Geometry: final body of the model. Coordinates: model frame, mm. A direction names the side the tool comes from. Give positions to 0.01 mm unless a question says otherwise; leave off trailing zeros. Order: outer loops, then holes, each group sorted by start corner. A loop starts at its lowest first (then second) coordinate and runs counter-clockwise, first axis right, second up. Notation, with made-up numbers: (42, -27.5) -> (66, -27.5) arc R35 ccw to (66, 10.5) -> close; hole circle Ø11 at (-1, 56.25). An arc over 180 degrees is marked (long way). One line per question, with ' | ' between items.
from build123d import *

# Parameters (mm, degrees)
BOSS_EXTRUDE1_DEPTH = 6.5
SKETCH2_R           = 12.5
BOSS_EXTRUDE2_DEPTH = 10.668
SKETCH3_R           = 10.5
BOSS_EXTRUDE3_DEPTH = 7
SKETCH4_R           = 7
BOSS_EXTRUDE4_DEPTH = 3


with BuildPart() as part:
    # Sketch1 → Boss-Extrude1 (new body)
    with BuildSketch(Plane.XY):
        with BuildLine():
            Line((-20.845394737, 3.828448545), (-5.427631579, 11.260142781))
            ThreePointArc((-5.427631579, 11.260142781), (0, 12.5), (5.427631579, 11.260142781))
            Line((5.427631579, 11.260142781), (20.845394737, 3.828448545))
            ThreePointArc((20.845394737, 3.828448545), (23.25, 0), (20.845394737, -3.828448545))
            Line((20.845394737, -3.828448545), (5.427631579, -11.260142781))
            ThreePointArc((5.427631579, -11.260142781), (0, -12.5), (-5.427631579, -11.260142781))
            Line((-5.427631579, -11.260142781), (-20.845394737, -3.828448545))
            ThreePointArc((-20.845394737, -3.828448545), (-23.25, 0), (-20.845394737, 3.828448545))
        make_face()
    extrude(amount=BOSS_EXTRUDE1_DEPTH)

    # Sketch2 → Boss-Extrude2 (add)
    with BuildSketch(Plane.XY.offset(6.5)):
        Circle(SKETCH2_R)
    extrude(amount=BOSS_EXTRUDE2_DEPTH)

    # Sketch3 → Boss-Extrude3 (add)
    with BuildSketch(Plane.XY.offset(17.168)):
        Circle(SKETCH3_R)
    extrude(amount=BOSS_EXTRUDE3_DEPTH)

    # Sketch4 → Boss-Extrude4 (add)
    with BuildSketch(Plane.XY.offset(24.168)):
        Circle(SKETCH4_R)
    extrude(amount=BOSS_EXTRUDE4_DEPTH)


solid = part.part
1) Section C-C on z = 4. Return loops of the section in (x, y), plus the area to 3 significant figures.
Check result:
outline: (-20.85, -3.83) -> (-5.43, -11.26) arc R12.5 ccw to (5.43, -11.26) -> (20.85, -3.83) arc R4.25 ccw to (20.85, 3.83) -> (5.43, 11.26) arc R12.5 ccw to (-5.43, 11.26) -> (-20.85, 3.83) arc R4.25 ccw to start | area: 754 mm^2
2) Set-up query: faces 1 (the flat face through (-13.029, -7.596, 3.204)), 2 (the cylindrical face through (10, 3.2, 20.6)). Return all of +Z, -Z, +X, -X, +Y, -Y with unobstructed straight access to the full face (end or side cutting, diameter ignored); none if empty.
Check result:
face 1: +Z, -Z, -X, -Y | face 2: +Z
3) Section D-D on y = 6.5. Return loops of the section in (x, z), plus the area to 3 significant figures.
Check result:
outline: (-15.3, 0) -> (15.3, 0) -> (15.3, 6.5) -> (10.68, 6.5) -> (10.68, 17.17) -> (8.25, 17.17) -> (8.25, 24.17) -> (2.6, 24.17) -> (2.6, 27.17) -> (-2.6, 27.17) -> (-2.6, 24.17) -> (-8.25, 24.17) -> (-8.25, 17.17) -> (-10.68, 17.17) -> (-10.68, 6.5) -> (-15.3, 6.5) -> close | area: 558 mm^2
4) Section A-A on x = 0. Return loops of the section in (y, z).
Check result:
outline: (-12.5, 0) -> (12.5, 0) -> (12.5, 17.17) -> (10.5, 17.17) -> (10.5, 24.17) -> (7, 24.17) -> (7, 27.17) -> (-7, 27.17) -> (-7, 24.17) -> (-10.5, 24.17) -> (-10.5, 17.17) -> (-12.5, 17.17) -> close
5) Section B-B on y = 0. Return loops of the section in (x, z), plus the area to 3 significant figures.
Check result:
outline: (-23.25, 0) -> (23.25, 0) -> (23.25, 6.5) -> (12.5, 6.5) -> (12.5, 17.17) -> (10.5, 17.17) -> (10.5, 24.17) -> (7, 24.17) -> (7, 27.17) -> (-7, 27.17) -> (-7, 24.17) -> (-10.5, 24.17) -> (-10.5, 17.17) -> (-12.5, 17.17) -> (-12.5, 6.5) -> (-23.25, 6.5) -> close | area: 758 mm^2
6) Material intervals for probe 1 along Z at (x, y) = (-6, -7.5); probe 2 along Z at (x, y) = (15, -0.75); probe 3 along Y at (x, z) = (-2, 16), sorted ascending. Write a range as from..to.
Check result:
probe 1: z = 0..24.17 | probe 2: z = 0..6.5 | probe 3: y = -12.34..12.34
7) Contact query for flat-ended pins moving along their axis: pin 1 Ø1 at (y, z) = (-9, 6.5) entering from -X; pin 2 Ø1.5 at (x, y) = (9.5, 2.5) entering from +Z; pin 3 Ø5 at (x, y) = (-11, -8.5) entering from +Z; pin 4 Ø14.5 at (x, y) = (-11, 3) entering from +Z. Output: stop coordinate, or through.
Check result:
pin 1: stops at x = -11.15 | pin 2: stops at z = 24.17 | pin 3: stops at z = 17.17 | pin 4: stops at z = 27.17
8) Pull-direction query (Z, two-part tool) for faces 3 (the flat face through (13.029, 7.596, 3.204)), 4 (the flat face through (2, -7, 24.168)), 5 (the flat face through (0, 0, 0)); classes: +Z half, -Z half, draft (parallel to the pull), parting line (faces both ways), or undercut.
Check result:
face 3: draft | face 4: +Z half | face 5: -Z half
